from build123d import *

# Parameters (mm, degrees)
ESQUISSE1_W             = 18
ESQUISSE1_H             = 30
BOSS_EXTRU_1_DEPTH      = 8.1
ESQUISSE3_R             = 1
ENL_V_MAT_EXTRU_1_DEPTH = 36.911140333
CONG_1_R                = 2.5


with BuildPart() as part:
    # Esquisse1 → Boss.-Extru.1 (new body)
    with BuildSketch(Plane.XY):
        with Locations((9, 15)):
            Rectangle(ESQUISSE1_W, ESQUISSE1_H)
    extrude(amount=BOSS_EXTRU_1_DEPTH)

    # Esquisse3 → Enlèv. mat.-Extru.1 (cut, through all)
    with BuildSketch(Plane.XY.offset(8.1)):
        with Locations((2.5, 26.2)):
            Circle(ESQUISSE3_R)
        with Locations((2.5, 9.2)):
            Circle(ESQUISSE3_R)
    extrude(amount=-ENL_V_MAT_EXTRU_1_DEPTH, mode=Mode.SUBTRACT)

    # Congé1
    cong_1_edges = [part.edges().sort_by_distance(p)[0] for p in [
        (0, 30, 4.05),
    ]]
    fillet(cong_1_edges, radius=CONG_1_R)


solid = part.part
CAD build for the part. Positions are in the model's coordinates, mm. Give positions to 0.01 mm unless a question says otherwise; leave off trailing zeros. Order: outer loops, then holes, each group sorted by start corner. A loop starts at its lowest first (then second) coordinate and runs counter-clockwise, first axis right, second up. Notation, with made-up numbers: (-40, -35) -> (-29, -35) arc R28 ccw to (-29, -16) -> close; hole circle Ø8 at (17, 7). An arc over 180 degrees is marked (long way). Return JSON: item names as keys, results as strings.
Q1. Mould opens along X. For faces 1 (the face through (9, 0, 4)), 2 (the face through (0, 14, 4)), 3 (the face through (18, 15, 4)), 4 (the face through (2.37, 10.19, 4.11)) say: pulls with the +X half, pulls with the -X half, needs draft (parallel to the pull), parting line crosses it, or undercut.
Working result:
{"face 1": "needs draft", "face 2": "pulls with the -X half", "face 3": "pulls with the +X half", "face 4": "undercut"}
Q2. Drill centre lines: line 1 (Y direction, x = 2.5, z = 4); line 2 (Y direction, x = 1.75, z = 0.5); line 3 (X direction, y = 9.25, z = 0.75). Where is each one in solid material? Low to high.
Working result:
{"line 1": "0 to 8.2, 10.2 to 25.2, 27.2 to 30", "line 2": "0 to 8.54, 9.86 to 25.54, 26.86 to 29.88", "line 3": "0 to 1.5, 3.5 to 18"}
Q3. Saw through at A-A (y = 26.2). Write the cut outline in (x, z).
Working result:
{"outline": "(0, 0) -> (1.5, 0) -> (1.5, 8.1) -> (0, 8.1) -> close; (3.5, 0) -> (18, 0) -> (18, 8.1) -> (3.5, 8.1) -> close"}
